Check sheet for the modelled part. Datum: model origin and axes. Units: mm. Give positions to 0.01 mm unless a question says otherwise; leave off trailing zeros. Write each loop counter-clockwise with the first axis right and the second up, starting at its lowest first coordinate (ties: lowest second). Pieces come first, ordered by that corner, then holes. Notation, with made-up numbers: M 79.25,-11.5 L 83.25,-11.5 A22 ccw 83.25,3.5 Z; hole C -34.75,31 d6. An arc over 180 degrees is marked long. Write item = value, one per line. Start each with the question number.
1) Scan lines: L1, parallel to X at y = 6, z = 47.25 (3 decimals); L2, parallel to X at y = 9, z = -31.75 (3 decimals); L3, parallel to X at y = 2.75, z = 31.75 (3 decimals). Record each from-to range of solid material in increasing order.
2) Draft check along Z on faces 1 (the face through (-30.31, 6.26, -44.68)), 2 (the face through (27.39, 6.26, -33.04)), 3 (the face through (0, 6, -57.15)), 4 (the face through (0, 6, 57.15)). Enter one of: pulls with the +Z half, pulls with the -Z half, needs draft (parallel to the pull), parting line crosses it, or undercut.
3) Gauge pin test, flat ends, axial feed: pin 1 (4 mm diameter, centred on x = -24.5, z = 29, fed in from -Y); pin 2 (2 mm diameter, centred on x = 28.575, z = -31.75, fed in from -Y). Record the tip position at first contact, or that the pin passes through.
4) Sectioned sample at A-A, the plane x = 0. Record the cut outline in (y, z).
5) Sectioned sample at B-B, the plane z = 16.25. Record the cut outline in (x, y) (3 decimals), then the cut area to 3 significant figures.
6) Sectioned sample at C-C, the plane y = 5.75. Count the separate pieces of the cut face and the enclosed holes in it, then the cut area to 3 significant figures.
Autodesk Inventor part; units mm, degrees
ref_plane "YZ Plane" through (0, 0, 0) normal (1, 0, 0) x (0, 1, 0)
ref_plane "XZ Plane" through (0, 0, 0) normal (0, 1, 0) x (-1, 0, 0)
ref_plane "XY Plane" through (0, 0, 0) normal (0, 0, 1) x (1, 0, 0)
sketch "Sketch1" plane through (0, 0, 0) normal (0, 1, 0) x (-1, 0, 0)
  line L0 (-34.925, -57.15) -> (34.925, -57.15)
  line L1 (34.925, -57.15) -> (34.925, 57.15)
  line L2 (34.925, 57.15) -> (-34.925, 57.15)
  line L3 (-34.925, 57.15) -> (-34.925, -57.15)
  line L4 (-34.925, -57.15) -> (34.925, 57.15) construction
  line L5 (34.925, -57.15) -> (-34.925, 57.15) construction
  point P0 (0, 0)
  dimension "d0" = 69.85
  dimension "d1" = 114.3
extrude "Extrusion1" add sketch "Sketch1" along normal blind 12.7
sketch "Sketch2" plane through (0, 12.7, 0) normal (0, 1, 0) x (1, 0, 0)
  line L0 (0, 0) -> (0, -188.6697)
  line L1 (43.5518, -31.75) -> (-58.772, -31.75)
  line L2 (52.9625, 0) -> (-57.3554, 0)
  line L3 (-34.925, -57.15) -> (34.925, -57.15)
  point P0 (15.494, -47.25)
  point P1 (15.494, -16.25)
  point P2 (-15.494, -47.25)
  point P3 (-15.494, -16.25)
  point P4 (0, -31.75)
  dimension "d7" = 31
  dimension "d8" = 30.988
  dimension "d46" = 25.4
hole "Hole1" at (15.494, 12.7, 47.25) at (15.494, 12.7, 16.25) at (-15.494, 12.7, 16.25) at (-15.494, 12.7, 47.25) direction (0, -1, 0) diameter 3.5 end through all
sketch "Sketch4" plane through (0, 12.7, 0) normal (0, 1, 0) x (1, 0, 0)
  circle A0 centre (15.494, -16.25) radius 1.75
  circle A1 centre (-15.494, -47.25) radius 1.75
  line L0 (15.494, -16.25) -> (-15.494, -47.25)
  circle A2 centre (-15.494, -16.25) radius 1.75
  circle A3 centre (15.494, -47.25) radius 1.75
  line L1 (-15.494, -16.25) -> (15.494, -47.25)
  point P0 (0, 0)
  point P1 (0, -31.75)
hole "Hole2" at (0, 12.7, 31.75) direction (0, -1, 0) diameter 10 end through all
sketch "Sketch6" plane through (0, 12.7, 0) normal (0, 1, 0) x (1, 0, 0)
  line L0 (0, -77.2056) -> (0, 91.7239)
  line L1 (-28.575, 6.35) -> (-28.575, 44.45)
  line L2 (-34.925, 57.15) -> (-34.925, -57.15)
  line L3 (-34.925, 0) -> (-34.925, 57.15)
  line L4 (28.575, 6.35) -> (28.575, 44.45)
  line L5 (-64.5272, 0) -> (76.1693, 0)
  line L6 (34.925, 57.15) -> (-34.925, 57.15)
  line L7 (34.925, 57.15) -> (-34.925, 57.15)
  point P0 (0, 0)
  point P1 (-28.575, 19.05)
  point P2 (-28.575, 31.75)
  point P3 (28.575, 19.05)
  point P4 (28.575, 31.75)
  dimension "d29" = 12.7
  dimension "d30" = 12.7
  dimension "d31" = 12.7
  dimension "d34" = 6.35
  dimension "d44" = 12.7
hole "Hole3" at (-28.575, 12.7, -6.35) at (-28.575, 12.7, -19.05) at (-28.575, 12.7, -31.75) at (-28.575, 12.7, -44.45) at (28.575, 12.7, -44.45) at (28.575, 12.7, -31.75) at (28.575, 12.7, -19.05) at (28.575, 12.7, -6.35) direction (0, -1, 0) diameter 3.5 end through all
properties part number "Lead_Screw_Fixture_Base"
Data:
q1.L1 = -34.925 to -17.244, -13.744 to 13.744, 17.244 to 34.925
q1.L2 = -34.925 to -30.325, -26.825 to 26.825, 30.325 to 34.925
q1.L3 = -34.925 to -5, 5 to 34.925
q2.face_1 = undercut
q2.face_2 = undercut
q2.face_3 = pulls with the -Z half
q2.face_4 = pulls with the +Z half
q3.pin_1 = 0
q3.pin_2 = through
q4.outline = M 0,-57.15 L 12.7,-57.15 L 12.7,26.75 L 0,26.75 Z; M 0,36.75 L 12.7,36.75 L 12.7,57.15 L 0,57.15 Z
q5.outline = M -34.925,0 L -17.244,0 L -17.244,12.7 L -34.925,12.7 Z; M -13.744,0 L 13.744,0 L 13.744,12.7 L -13.744,12.7 Z; M 17.244,0 L 34.925,0 L 34.925,12.7 L 17.244,12.7 Z
q5.area = 798 mm2
q6.separate_pieces = 1
q6.enclosed_holes = 13
q6.area = 7,790 mm2
